For this review, take the finished solid that the model builds, in its own axes (mm). Round coordinates to 2 decimals unless told otherwise and drop trailing zeros. Loops run counter-clockwise (first coordinate to the right, second up) from the corner with the lowest first, then second, coordinate; pieces in that order, holes last. Notation, with made-up numbers: M -13,0 L -1,0 A16 ccw -1,29 Z; hole C -21,-27 d3. An arc over 180 degrees is marked long. One line per question, with ' | ' between items. Start each with the question number.
1) For probe 1 along Y at (x, z) = (631, 7.75); probe 2 along X at (y, z) = (255.5, 16.75); probe 3 along X at (y, z) = (225, 6.25), list the stretches that pass through material, from the lowest coordinate up. Write a range as from..to.
2) We need section C-C (z = 9). Give the boundary of the cut face in (x, y), and give its area (3 significant figures).
3) We need section B-B (y = 118). Give the boundary of the cut face in (x, z), and give its area (3 significant figures).
4) We need section A-A (x = -2). Give the boundary of the cut face in (y, z), and give its area (3 significant figures).
5) For pin 1 Ø5 at (y, z) = (309.5, 21.5) entering from +X; pin 2 Ø2 at (y, z) = (140.5, 15) entering from +X; pin 3 Ø12.5 at (y, z) = (82.5, 18.5) entering from +X, all flat-tipped, find the tip position at first contact; note any pin that passes through.
6) We need section D-D (y = -511.5). Give the boundary of the cut face in (x, z), and give its area (3 significant figures).
```python
from build123d import *

# Parameters (mm, degrees)
F0_W     = 1875
F0_H     = 660
F1_DEPTH = 25


with BuildPart() as f1:
    # F0 (on Top) → F1 (new body)
    with BuildSketch(Plane.XY):
        with BuildLine():
            Line((1037.5, 430), (-1037.5, 430))
            ThreePointArc((-1037.5, 430), (-1237.5, -100), (-1037.5, -630))
            Line((-1037.5, -630), (1037.5, -630))
            ThreePointArc((1037.5, -630), (1237.5, -100), (1037.5, 430))
        make_face()
        Rectangle(F0_W, F0_H, mode=Mode.SUBTRACT)
    extrude(amount=F1_DEPTH)


solid = f1.part
```
Answers below:
1) probe 1: -630..-330, 330..430 | probe 2: -1154.43..-937.5, 937.5..1154.43 | probe 3: -1168.72..-937.5, 937.5..1168.72
2) outline: M -1037.5,-630 L 1037.5,-630 A802.25 ccw 1037.5,430 L -1037.5,430 A802.25 ccw Z; hole M -937.5,-330 L 937.5,-330 L 937.5,330 L -937.5,330 Z | area: 1,250,000 mm^2
3) outline: M -1207.31,0 L -937.5,0 L -937.5,25 L -1207.31,25 Z; M 937.5,0 L 1207.31,0 L 1207.31,25 L 937.5,25 Z | area: 13,500 mm^2
4) outline: M -630,0 L -330,0 L -330,25 L -630,25 Z; M 330,0 L 430,0 L 430,25 L 330,25 Z | area: 10,000 mm^2
5) pin 1: x = 1126.59 | pin 2: x = 1200.92 | pin 3: x = 1217.9
6) outline: M -1123.92,0 L 1123.92,0 L 1123.92,25 L -1123.92,25 Z | area: 56,200 mm^2
